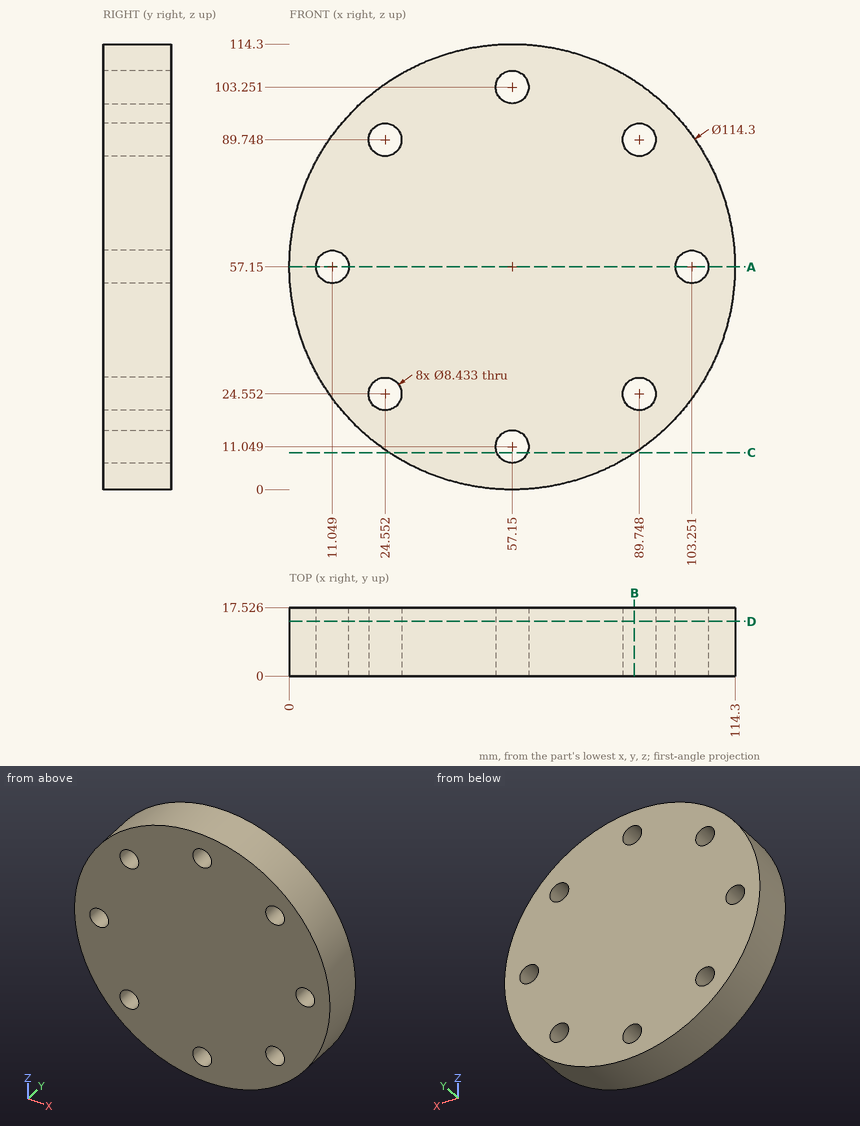
Geometry check sheet. Reference: drawing and pictorial views, mm from the part's lowest x, y, z. Give positions to 0.01 mm unless a question says otherwise; leave off trailing zeros. Order: outer loops, then holes, each group sorted by start corner. A loop starts at its lowest first (then second) coordinate and runs counter-clockwise, first axis right, second up. Notation, with made-up numbers: M 68.5,21.25 L 120.5,21.25 A30 ccw 120.5,47.25 Z; hole C -19.5,83.5 d4. An arc over 180 degrees is marked long. Answer in a Markdown table with one row per item.
1) Cross-section at B-B, the plane x = 88.5. Enter the section's corners in (y, z).
Filled sheet:
| item | result |
|---|---|
| outline | M 0,9.37 L 17.53,9.37 L 17.53,20.52 L 0,20.52 Z; M 0,28.58 L 17.53,28.58 L 17.53,85.72 L 0,85.72 Z; M 0,93.78 L 17.53,93.78 L 17.53,104.93 L 0,104.93 Z |
2) Gauge pin test, flat ends, axial feed: P1, Ø6, axis at y = 9, z = 30, coming from the -X side; P2, Ø10, axis at x = 80, y = 10.5, coming from the +Z side; P3, Ø3, axis at y = 9, z = 41, coming from the +X side. Record the tip position at first contact, or that the pin passes through.
Filled sheet:
| item | result |
|---|---|
| P1 | stops at x = 5.35 |
| P2 | stops at z = 111.44 |
| P3 | stops at x = 112.39 |
3) Cross-section at A-A, the plane z = 57.15. Enter the section's corners in (x, y) (1 decimal).
Filled sheet:
| item | result |
|---|---|
| outline | M 0,0 L 6.8,0 L 6.8,17.5 L 0,17.5 Z; M 15.3,0 L 99,0 L 99,17.5 L 15.3,17.5 Z; M 107.5,0 L 114.3,0 L 114.3,17.5 L 107.5,17.5 Z |
4) Cross-section at D-D, the plane y = 14. Count the separate pieces of the cut face and the enclosed holes in it, plus the area to 3 significant figures.
Filled sheet:
| item | result |
|---|---|
| separate pieces | 1 |
| enclosed holes | 8 |
| area | 9,810 mm2 |
5) Cross-section at C-C, the plane z = 9.5. Enter the section's corners in (x, y).
Filled sheet:
| item | result |
|---|---|
| outline | M 25.6,0 L 53.23,0 L 53.23,17.53 L 25.6,17.53 Z; M 61.07,0 L 88.7,0 L 88.7,17.53 L 61.07,17.53 Z |
6) Thickness scan on L1, parallel to X at y = 5.75, z = 24.5 (1 decimal); L2, parallel to Z at x = 25, y = 11.25 (1 decimal); L3, parallel to X at y = 12, z = 26 (1 decimal). Record the ranges inside material, lowest first. Write a range as [from, to].
Filled sheet:
| item | result |
|---|---|
| L1 | x = [10.2, 20.3], [28.8, 85.5], [94, 104.1] |
| L2 | z = [9.9, 20.4], [28.7, 85.6], [93.9, 104.4] |
| L3 | x = [9.2, 20.6], [28.5, 85.8], [93.7, 105.1] |
